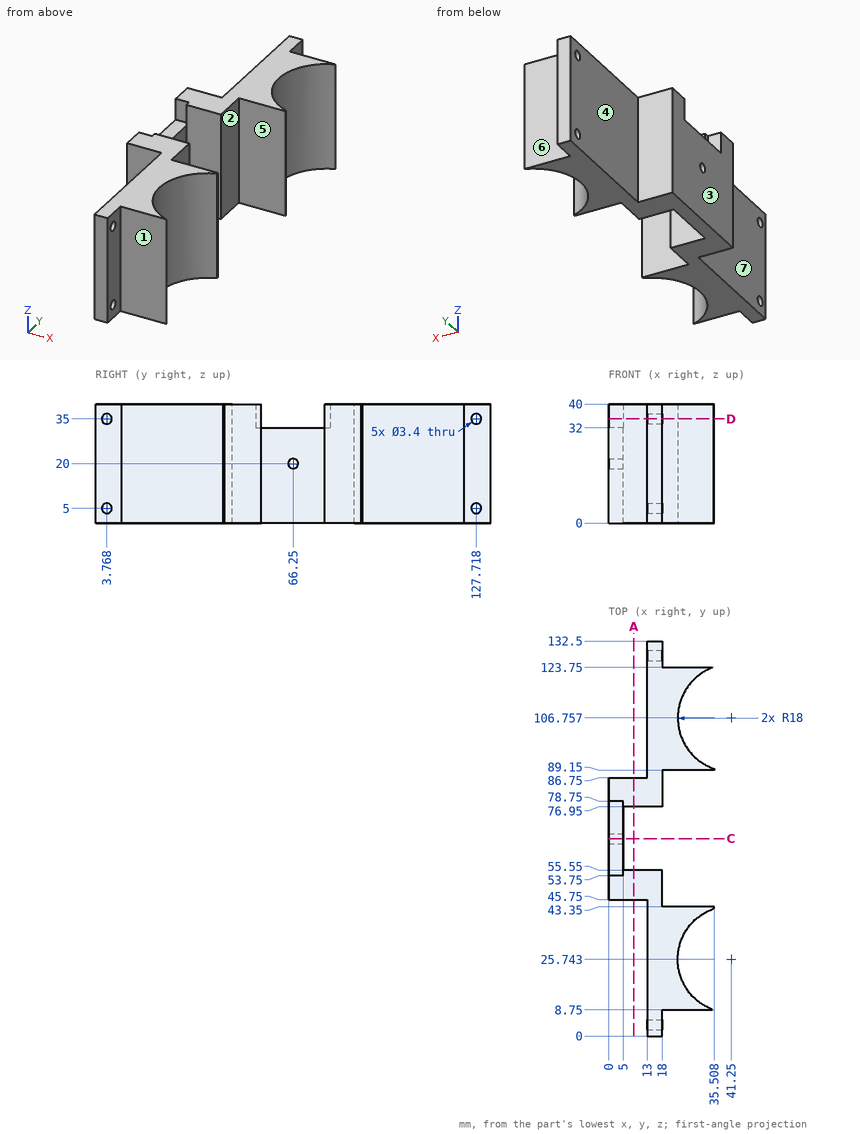
Could you check a few things on this drawing? It's one solid part, dimensions in mm from its lowest x, y, z. A direction names the side the tool comes from. Give positions to 0.01 mm unless a question says otherwise; leave off trailing zeros. Loops run counter-clockwise (first coordinate to the right, second up) from the corner with the lowest first, then second, coordinate; pieces in that order, holes last. Notation, with made-up numbers: M 68.5,-24.75 L 77.5,-24.75 A26 cw 77.5,8.25 Z; hole C -4.5,-17.75 d9. An arc over 180 degrees is marked long. Return JSON: item names as keys, results as strings.
Item 1: Imagine slicing it at A-A on x = 8.5. List the corners of the cut face in (y, z) for me, then the cut area to 3 significant figures.
A:
{"outline": "M 45.75,0 L 55.55,0 L 55.55,40 L 45.75,40 Z; M 76.95,0 L 86.75,0 L 86.75,40 L 76.95,40 Z", "area": "784 mm^2"}
Item 2: I'm going to push flat-ended pins straight in: pin 1 Ø1.5 at (x, z) = (9, 4.5) entering from -Y; pin 2 Ø2 at (x, y) = (5, 59) entering from +Z; pin 3 Ø12 at (y, z) = (22.5, 10) entering from -X. Where does each tip first touch, or does it pass through?
A:
{"pin 1": "stops at y = 45.75", "pin 2": "stops at z = 32", "pin 3": "stops at x = 13"}
Item 3: On a 3-axis mill with a long thin cutter (end or side, diameter ignored), from which of +Z, -Z, +X, -X, +Y, -Y can I reach the whole of each face in a straight line? I mean the marked faces 4, 5, 6 and 7. Say none if no direction works.
A:
{"face 4": "+Z, -Z, -X, +Y", "face 5": "+Z, -Z, +X", "face 6": "+Z, -Z, +X, +Y", "face 7": "+Z, -Z, -X, -Y"}
Item 4: Imagine slicing it at C-C on y = 66.25. List the corners of the cut face in (x, z) for me.
A:
{"outline": "M 0,0 L 5,0 L 5,18.3 L 0,18.3 Z; M 0,21.7 L 5,21.7 L 5,32 L 0,32 Z"}
Item 5: Thinking about a two-plate mould opening in Y: for the marked faces 1, 2 and 3, which applies, released by +Y, released by -Y, zero draft, split by the parting line, or undercut?
A:
{"face 1": "released by -Y", "face 2": "undercut", "face 3": "zero draft"}
Item 6: Please list where these lines run through material, in increasing order: line 1 (Y direction, x = 15.2, z = 5); line 2 (Y direction, x = 10, z = 16); line 3 (Y direction, x = 16.5, z = 26).
A:
{"line 1": "y = 0 to 2.07, 5.47 to 55.55, 76.95 to 126.02, 129.42 to 132.5", "line 2": "y = 45.75 to 55.55, 76.95 to 86.75", "line 3": "y = 0 to 55.55, 76.95 to 132.5"}
Item 7: Imagine slicing it at D-D on z = 35. State how many separate pieces and enclosed holes the cut face has, then the cut area to 3 significant figures.
A:
{"separate pieces": "4", "enclosed holes": "0", "area": "1,360 mm^2"}
